Could you check a few things on this model? Use its own coordinates, in mm. A direction names the side the tool comes from. Coordinates: 2 decimals unless noted, no trailing zeros. Loops run counter-clockwise (first coordinate to the right, second up) from the corner with the lowest first, then second, coordinate; pieces in that order, holes last.
from build123d import *

# Parameters (mm, degrees)
BOSS_EXTRU_1_DEPTH        = 3
BOSS_EXTRU_1_DEPTH_BACK   = 3
ESQUISSE1_W               = 4
ESQUISSE1_H               = 4
BOSS_EXTRU_1_2_DEPTH      = 3
BOSS_EXTRU_1_2_DEPTH_BACK = 3
BOSS_EXTRU_2_DEPTH        = 1.5
BOSS_EXTRU_2_DEPTH_BACK   = 1.5
ESQUISSE4_R               = 1
ENL_V_MAT_EXTRU_1_DEPTH   = 21.5
ENL_V_MAT_EXTRU_2_DEPTH   = 21.5


with BuildPart() as part:
    # Esquisse1 → Boss.-Extru.1 (new, two sides: drawn at the far end of the back side and taken through both)
    with BuildSketch(Plane(origin=(0, 0, 0), x_dir=(1, 0, 0), z_dir=(0, 1, 0)).offset(-BOSS_EXTRU_1_DEPTH_BACK)):
        with Locations((0, 20.5)):
            Rectangle(ESQUISSE1_W, ESQUISSE1_H)
    extrude(amount=BOSS_EXTRU_1_DEPTH + BOSS_EXTRU_1_DEPTH_BACK)



with BuildPart() as body_2:
    # Esquisse1 → Boss.-Extru.1 2 (new, two sides: drawn at the far end of the back side and taken through both)
    with BuildSketch(Plane(origin=(0, 0, 0), x_dir=(1, 0, 0), z_dir=(0, 1, 0)).offset(-BOSS_EXTRU_1_2_DEPTH_BACK)):
        with Locations((0, -20.5)):
            Rectangle(ESQUISSE1_W, ESQUISSE1_H)
    extrude(amount=BOSS_EXTRU_1_2_DEPTH + BOSS_EXTRU_1_2_DEPTH_BACK)


with BuildPart() as part_1:
    add(part.part)

    add(body_2.part)  # Boss.-Extru.2 merges body 2
    # Esquisse3 → Boss.-Extru.2 (add, two sides: drawn at the far end of the back side and taken through both)
    with BuildSketch(Plane(origin=(0, 0, 0), x_dir=(1, 0, 0), z_dir=(0, 1, 0)).offset(-BOSS_EXTRU_2_DEPTH_BACK)):
        with BuildLine():
            Line((-2, 18.571568884), (1.93, 18.571568884))
            add(Edge.make_bspline(
                [(1.93, 18.571568884), (2.088145302, 18.144214449), (2.536201665, 18.035775419)],
                knots=[0, 0, 0, 1, 1, 1], degree=2))
            Line((2.536201665, 18.035775419), (11.300625785, 18.035775419))
            Line((11.300625785, 18.035775419), (11.300625785, -18.091491534))
            Line((11.300625785, -18.091491534), (2.536201665, -18.091491534))
            add(Edge.make_bspline(
                [(2.536201665, -18.091491534), (2.088145302, -18.199930564), (1.93, -18.627284999)],
                knots=[0, 0, 0, 1, 1, 1], degree=2))
            Line((1.93, -18.627284999), (-2, -18.627284999))
            Line((-2, -18.627284999), (-2, 18.571568884))
        make_face()
    extrude(amount=BOSS_EXTRU_2_DEPTH + BOSS_EXTRU_2_DEPTH_BACK)

    # Esquisse4 → Enl_v. mat.-Extru.1 (cut)
    with BuildSketch(Plane(origin=(0, 1.5, 0), x_dir=(1, 0, 0), z_dir=(0, 1, 0))):
        with Locations(Location((9.75, 9.645867946, 0), (0, 0, 270))):
            Circle(ESQUISSE4_R)
        with Locations(Location((9.75, -9.654132054, 0), (0, 0, 90))):
            Circle(ESQUISSE4_R)
    extrude(amount=-ENL_V_MAT_EXTRU_1_DEPTH, mode=Mode.SUBTRACT)

    # Esquisse5 → Enl_v. mat.-Extru.2 (cut)
    with BuildSketch(Plane(origin=(2, 0, 0), x_dir=(0, 0, -1), z_dir=(1, 0, 0))):
        with BuildLine():
            Line((-19.4, 1.4), (-19.4, -1.4))
            ThreePointArc((-19.4, -1.4), (-20.5, -2.5), (-21.6, -1.4))
            Line((-21.6, -1.4), (-21.6, 1.4))
            ThreePointArc((-21.6, 1.4), (-20.5, 2.5), (-19.4, 1.4))
        make_face()
        with BuildLine():
            Line((19.4, 1.4), (19.4, -1.4))
            ThreePointArc((19.4, -1.4), (20.5, -2.5), (21.6, -1.4))
            Line((21.6, -1.4), (21.6, 1.4))
            ThreePointArc((21.6, 1.4), (20.5, 2.5), (19.4, 1.4))
        make_face()
    extrude(amount=-ENL_V_MAT_EXTRU_2_DEPTH, mode=Mode.SUBTRACT)


solid = part_1.part
(1) Imagine slicing it at B-B, the plane x = 1.5. Write out the boundary of the cut face in (y, z), and give its area (3 significant figures).
Answers:
outline: (-3, -22.5) - (3, -22.5) - (3, -18.5) - (1.5, -18.5) - (1.5, 18.5) - (3, 18.5) - (3, 22.5) - (-3, 22.5) - (-3, 18.5) - (-1.5, 18.5) - (-1.5, -18.5) - (-3, -18.5) - close; hole (-1.4, -21.6) - (1.4, -21.6) arc R1.1 ccw to (1.4, -19.4) - (-1.4, -19.4) arc R1.1 ccw to start; hole (-1.4, 19.4) - (1.4, 19.4) arc R1.1 ccw to (1.4, 21.6) - (-1.4, 21.6) arc R1.1 ccw to start
area: 139 mm2
(2) Which directions (+Z, -Z, +X, -X, +Y, -Y) give clear straight access to the entire face, cutting with the end or side of a thin tool? Please do faces 5 (the face through (7, 0, -18.036)), 6 (the face through (2, 0, 22)), 7 (the face through (0, 0, -21.6)), 8 (the face through (5, -1.5, 0)), 9 (the face through (5, 1.5, 0)).
Answers:
face 5: -Z, +X, +Y, -Y
face 6: +Z, +X, +Y, -Y
face 7: +X, -X
face 8: +X, -X, -Y
face 9: +X, -X, +Y
(3) Imagine slicing it at A-A, the plane z = -20.5. Write out the boundary of the cut face in (x, y), and give its area (3 significant figures).
Answers:
outline: (-2, -3) - (2, -3) - (2, -2.5) - (-2, -2.5) - close; (-2, 2.5) - (2, 2.5) - (2, 3) - (-2, 3) - close
area: 4.00 mm2
(4) For pin 1 (2 mm diameter, centred on x = 1, z = -8, fed in from +Y); pin 2 (1.6 mm diameter, centred on x = 9.75, z = 9.65, fed in from -Y); pin 3 (1.5 mm diameter, centred on x = 6.5, y = -0.5, fed in from +Z); pin 4 (2 mm diameter, centred on y = -1, z = 21.5, fed in from +X), each with a flat end and sliding along its axis, tell me the tip position at first contact or that it passes through.
Answers:
pin 1: stops at y = 1.5
pin 2: passes through
pin 3: stops at z = 18.09
pin 4: stops at x = 2
(5) We'd pull the mould along X, two halves only. Please class faces 1 (the face through (0, 0, 21.6)), 2 (the face through (10.05, 0.02, -8.69)), 3 (the face through (8.759, 0.021, 9.784)), 4 (the face through (11.301, 0, 0)): +X half, -X half, draft (parallel to the pull), parting line (faces both ways), or undercut.
Answers:
face 1: draft
face 2: undercut
face 3: undercut
face 4: +X half
(6) Imagine slicing it at D-D, the plane x = 6.25. Write out the boundary of the cut face in (y, z).
Answers:
outline: (-1.5, -18.04) - (1.5, -18.04) - (1.5, 18.09) - (-1.5, 18.09) - close
(7) I need wall thicknesses on probe 1 along Z at (x, y) = (-1, -1.25); probe 2 along Z at (x, y) = (9.25, 0.25); probe 3 along Y at (x, z) = (0, -7). Which ranges of each line are inside material? Lowest first, please.
Answers:
probe 1: z = -22.5 to -21.6, -19.4 to 19.4, 21.6 to 22.5
probe 2: z = -18.04 to -10.51, -8.78 to 8.79, 10.52 to 18.09
probe 3: y = -1.5 to 1.5
(8) Imagine slicing it at C-C, the plane y = 0. State how many separate pieces and enclosed holes the cut face has, and give its area (3 significant figures).
Answers:
separate pieces: 3
enclosed holes: 2
area: 492 mm2
